Check sheet for the modelled part. Datum: model origin and axes. Units: mm. A direction names the side the tool comes from. Give positions to 0.01 mm unless a question says otherwise; leave off trailing zeros. Order: outer loops, then holes, each group sorted by start corner. A loop starts at its lowest first (then second) coordinate and runs counter-clockwise, first axis right, second up.
Item 1: Material ranges on line 1 along Y through (x, z) = (6.25, 42); line 2 along X through (y, z) = (65, 62); line 3 along Z through (x, y) = (7.5, 85.5), recorded low to high.
Item 2: Gauge pin test, flat end, axial feed: P1, Ø12, axis at y = 50, z = 18.5, coming from the -X side. Record the tip position at first contact, or that the pin passes through.
Item 3: Access from +Z, -Z, +X, -X, +Y, -Y to the whole of each face (thin tool, end or side, straight path). Record for faces 1 (the flat face through (12, 90, 53)), 2 (the flat face through (12, 94, 53)).
Item 4: Sectioned sample at A-A on x = 11.75. Record the boundary of the cut face in (y, z), and give its area (3 significant figures).
Item 5: Release check for a two-part mould opening along Z. For faces 3 (the flat face through (12, 48, 0)), 4 (the flat face through (12, 4, 53)), 5 (the flat face through (25, 46, 53)) record: released by +Z, released by -Z, zero draft, split by the parting line, or undercut.
Item 6: Sectioned sample at B-B on y = 45. Record the boundary of the cut face in (x, z).
from build123d import *

# Parameters (mm, degrees)
SKETCH_1_W      = 25
SKETCH_1_H      = 94
EXTRUDE_1_DEPTH = 108
SHELL_2_T       = 4


with BuildPart() as part:
    # 草图1 → 凸台-拉伸1 (new body)
    with BuildSketch(Plane.XY):
        with Locations((12.5, 47)):
            Rectangle(SKETCH_1_W, SKETCH_1_H)
    extrude(amount=EXTRUDE_1_DEPTH)

    # 抽壳2 (no face opened: a closed hollow body)
    add(offset(amount=-SHELL_2_T, mode=Mode.PRIVATE), mode=Mode.SUBTRACT)


solid = part.part
Report:
1. line 1: y = 0 to 4, 90 to 94
1. line 2: x = 0 to 4, 21 to 25
1. line 3: z = 0 to 4, 104 to 108
2. P1: stops at x = 0
3. face 1: none
3. face 2: +Z, -Z, +X, -X, +Y
4. outline: (0, 0) - (94, 0) - (94, 108) - (0, 108) - close; hole (4, 4) - (90, 4) - (90, 104) - (4, 104) - close
4. area: 1,550 mm2
5. face 3: released by -Z
5. face 4: undercut
5. face 5: zero draft
6. outline: (0, 0) - (25, 0) - (25, 108) - (0, 108) - close; hole (4, 4) - (21, 4) - (21, 104) - (4, 104) - close
